```python
from build123d import *

# Parameters (mm, degrees)
F0_W      = 20
F0_H      = 19
F1_DEPTH  = 6
F2_R      = 6.8
F3_DEPTH  = 0.8
F4_R      = 6
F5_DEPTH  = 3.2
F6_R      = 3.5
F7_DEPTH  = 2
F11_DEPTH = 9.5
F12_W     = 24
F12_H     = 5
F13_DEPTH = 9.5
F15_DEPTH = 5
F16_R     = 3.25
F17_DEPTH = 25
F18_W     = 26
F18_H     = 5
F19_DEPTH = 12.5


with BuildPart() as f1:
    # F0 (on Right) → F1 (new body)
    with BuildSketch(Plane.YZ):
        Rectangle(F0_W, F0_H)
    extrude(amount=F1_DEPTH)

    # F2 (on face) → F3 (cut)
    with BuildSketch(Plane.YZ.offset(6)):
        with Locations((0, -1)):
            Circle(F2_R)
    extrude(amount=-F3_DEPTH, mode=Mode.SUBTRACT)

    # F4 (on face) → F5 (cut)
    with BuildSketch(Plane.YZ.offset(5.2)):
        with Locations((0, -1)):
            Circle(F4_R)
    extrude(amount=-F5_DEPTH, mode=Mode.SUBTRACT)

    # F6 (on face) → F7 (cut, through all)
    with BuildSketch(Plane.YZ.offset(2)):
        with Locations((0, -1)):
            Circle(F6_R)
    extrude(amount=-F7_DEPTH, mode=Mode.SUBTRACT)


with BuildPart() as f9_1:
    # F9: instance of F1
    add(f1.part.mirror(Plane.YZ.offset(-16)))


with BuildPart() as f1_1:
    add(f1.part)

    add(f9_1.part)  # F11 merges F9_1
    # F10 (on Top) → F11 (join, symmetric)
    with BuildSketch(Plane.XY):
        with BuildLine():
            ThreePointArc((-32, 10), (-16, 18.8679622641), (0, 10))
            Line((0, 10), (6, 10))
            ThreePointArc((6, 10), (-16, 24.1660919472), (-38, 10))
            Line((-38, 10), (-32, 10))
        make_face()
    extrude(amount=F11_DEPTH, both=True)

    # F12 (on Top) → F13 (join, symmetric)
    with BuildSketch(Plane.XY):
        with Locations((-16, 17.0602197786)):
            Rectangle(F12_W, F12_H)
    extrude(amount=F13_DEPTH, both=True)

    # F14 (on face) → F15 (cut)
    with BuildSketch(Plane.XZ.offset(-14.5602197786)):
        Polygon((-18.8867513459, -5), (-13.1132486541, -5), (-10.2264973081, 0), (-13.1132486541, 5), (-18.8867513459, 5), (-21.7735026919, 0), align=None)
    extrude(amount=-F15_DEPTH, mode=Mode.SUBTRACT)

    # F16 (on face) → F17 (cut)
    with BuildSketch(Plane.XZ.offset(-19.5602197786)):
        with Locations((-15.9966088831, 0)):
            Circle(F16_R)
    extrude(amount=-F17_DEPTH, mode=Mode.SUBTRACT)

    # F18 (on Top) → F19 (cut, symmetric)
    with BuildSketch(Plane.XY):
        with Locations((-16, 25.0602197786)):
            Rectangle(F18_W, F18_H)
    extrude(amount=F19_DEPTH, both=True, mode=Mode.SUBTRACT)


solid = f1_1.part
```
The listing builds one solid part. Answer for the finished solid, in the listing's coordinates (mm). A direction names the side the tool comes from. Coordinates: 2 decimals unless noted, no trailing zeros. Write each loop counter-clockwise with the first axis right and the second up, starting at its lowest first coordinate (ties: lowest second). Pieces come first, ordered by that corner, then holes. Notation, with made-up numbers: (-6.5, 25) - (19.5, 25) arc R34 cw to (19.5, 60) - close; hole circle Ø10 at (1.5, 64). An arc over 180 degrees is marked (long way). Return JSON: item names as keys, results as strings. Group by question number.
Q1. The part is cut by section C-C on z = 7. Write down the section's boundary in (x, y), and give its area (3 significant figures).
Q2. Which of the six approach directions +Z, -Z, +X, -X, +Y, -Y give full straight-line access (tool end or side, diameter ignored) to faces 4 (the flat face through (-34, 3, -4)), 5 (the flat face through (-22, 14.56, 2)), 6 (the flat face through (-16.1, 19.56, 3.4))?
Q3. The part is cut by section D-D on x = -15.5. Write down the section's boundary in (y, z).
Q4. Flat-ended cylindrical pins translate along their axes: pin 1 Ø10 at (x, y) = (-6, 9) entering from +Z; pin 2 Ø4 at (x, z) = (-11.5, -1.5) entering from -Y; pin 3 Ø1.5 at (y, z) = (-6, -1) entering from +X; pin 4 Ø11 at (y, z) = (0, -1) entering from +X. Find the tip coordinate at first contact, or state that the pin passes through.
Q5. Find the intervals of material crossed by line 1 along Z through (x, y) = (-37.35, 0); line 2 along Z through (x, y) = (-33, 0); line 3 along X through (y, z) = (10, -7), in increasing order. Write a range as [from, to].
Q6. The part is cut by section A-A on y = 8. Write down the section's boundary in (x, z), and give its area (3 significant figures).
Q7. The part is cut by section B-B on y = 0. State how many separate pieces and enclosed holes the cut face has, and give its area (3 significant figures).
Q8. For a pull along Y with two mould halves and no side action, classify faces 1 (the flat face through (6, -5, 4)), 2 (the flat face through (-37.2, 4, -6)), 3 (the flat face through (-20, 22.56, 0)) as +Y half, -Y half, draft (parallel to the pull), parting line (faces both ways), or undercut.
Evaluation:
{
 "1": {"outline": "(-38, -10) - (-32, -10) - (-32, 10) arc R18.87 cw to (-28, 14.56) - (-4, 14.56) arc R18.87 cw to (0, 10) - (0, -10) - (6, -10) - (6, 10) arc R24.17 ccw to (-7.34, 22.56) - (-24.66, 22.56) arc R24.17 ccw to (-38, 10) - close", "area": "540 mm2"},
 "2": {"face 4": "-X", "face 5": "+Z, -Z, -Y", "face 6": "-Y"},
 "3": {"outline": "(14.56, -9.5) - (22.56, -9.5) - (22.56, -3.21) - (19.56, -3.21) - (19.56, -5) - (14.56, -5) - close; (14.56, 5) - (19.56, 5) - (19.56, 3.21) - (22.56, 3.21) - (22.56, 9.5) - (14.56, 9.5) - close"},
 "4": {"pin 1": "passes through", "pin 2": "stops at y = 14.56", "pin 3": "stops at x = 5.2", "pin 4": "stops at x = 2"},
 "5": {"line 1": "z = [-9.5, -7.8], [5.8, 9.5]", "line 2": "z = [-9.5, -4.5], [2.5, 9.5]", "line 3": "x = [-38, -32], [0, 6]"},
 "6": {"outline": "(-38, -9.5) - (-32, -9.5) - (-32, 9.5) - (-38, 9.5) - close; (0, -9.5) - (6, -9.5) - (6, 9.5) - (0, 9.5) - close", "area": "228 mm2"},
 "7": {"separate pieces": "4", "enclosed holes": "0", "area": "101 mm2"},
 "8": {"face 1": "draft", "face 2": "undercut", "face 3": "+Y half"}
}
